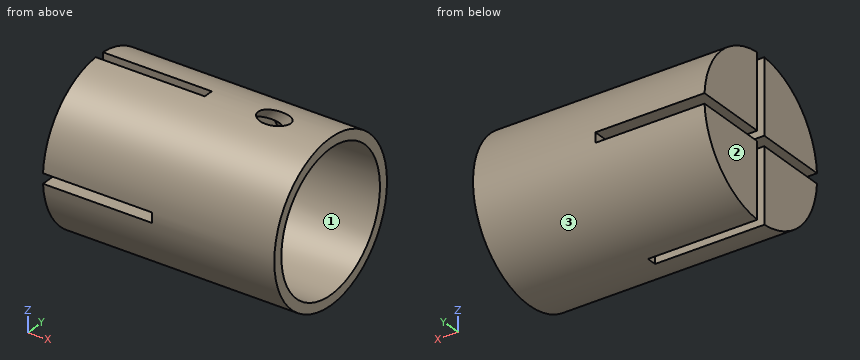
```python
from build123d import *

# Parameters (mm, degrees)
F2_W     = 36.676987372
F2_H     = 3.81
F2_W_2   = 3.81
F2_H_2   = 32.5926636749
F2_W_3   = 35.713012628
F2_H_3   = 39.7973363251
F3_DEPTH = 41.91
F6_R     = 4.445
F7_DEPTH = 76.708


with BuildPart() as f1:
    # F0 (on Front) → F1 (revolve)
    with BuildSketch(Plane.XZ):
        Polygon((-47.0309668349, 30.48), (-47.0309668349, 0), (3.7690331651, 0), (3.7690331651, 26.67), (41.8690331651, 26.67), (41.8690331651, 30.48), align=None)
    revolve(axis=Axis((6.2270945557, 0, 0), (1, 0, 0)))

    # F2 (on face) → F3 (cut)
    with BuildSketch(Plane(origin=(-47.0309668349, 0, 0), x_dir=(0, -1, 0), z_dir=(-1, 0, 0))):
        with Locations((-20.243493686, 0)):
            Rectangle(F2_W, F2_H)
        with Locations((0, 18.2013318375)):
            Rectangle(F2_W_2, F2_H_2)
        Rectangle(F2_W_2, F2_H)
        with Locations((19.761506314, 0)):
            Rectangle(F2_W_3, F2_H)
        with Locations((0, -21.8036681625)):
            Rectangle(F2_W_2, F2_H_3)
    extrude(amount=-F3_DEPTH, mode=Mode.SUBTRACT)

    # F6 (on line) → F7 (cut)
    with BuildSketch(Plane(origin=(66.1142536219, 0, 66.1142536219), x_dir=(0, -1, 0), z_dir=(-0.7071067812, 0, -0.7071067812))):
        with Locations((0, 7.1842048969)):
            Circle(F6_R)
    extrude(amount=F7_DEPTH, mode=Mode.SUBTRACT)


solid = f1.part
```
The model under review builds one solid part; all positions refer to its coordinate system, in mm. Face numbers are marked on the shaded views. Round coordinates to 2 decimals unless told otherwise and drop trailing zeros. Loops run counter-clockwise (first coordinate to the right, second up) from the corner with the lowest first, then second, coordinate; pieces in that order, holes last.
1) Consider section C-C on y = 0. State the section outline as (x, z) points, then the cut area to 3 significant figures.
Values follow:
outline: (-5.12, -30.48) - (41.87, -30.48) - (41.87, -26.67) - (3.77, -26.67) - (3.77, 19.98) - (3.65, 20.1) - (3.77, 20.22) - (3.77, 26.67) - (10.22, 26.67) - (14.03, 30.48) - (-5.12, 30.48) - close; (22.8, 26.67) - (41.87, 26.67) - (41.87, 30.48) - (26.61, 30.48) - close
area: 784 mm2
2) Consider section B-B on x = -11.5. State the section outline as (y, z) points (3 decimals), then the cut area to 3 significant figures.
Values follow:
outline: (-30.42, -1.905) arc R30.48 ccw to (-1.905, -30.42) - (-1.905, -1.905) - close; (-30.42, 1.905) - (-1.905, 1.905) - (-1.905, 30.42) arc R30.48 ccw to start; (1.905, -30.42) arc R30.48 ccw to (30.42, -1.905) - (1.905, -1.905) - close; (1.905, 1.905) - (30.42, 1.905) arc R30.48 ccw to (1.905, 30.42) - close
area: 2,470 mm2
3) Wall thickness on line 1 along Y through (x, z) = (25.5, 0); line 2 along X through (y, z) = (-10.5, -2); line 3 along Z through (x, y) = (18.5, 0): over which ranges is each line inside the solid? List them lowest first.
Values follow:
line 1: y = -30.48 to -26.67, 26.67 to 30.48
line 2: x = -47.03 to 3.77
line 3: z = -30.48 to -26.67
4) Consider section D-D on y = -20. State the section outline as (x, z) points (3 decimals), then the cut area to 3 significant figures.
Values follow:
outline: (-47.031, -23.001) - (41.869, -23.001) - (41.869, -17.643) - (3.769, -17.643) - (3.769, 17.643) - (41.869, 17.643) - (41.869, 23.001) - (-47.031, 23.001) - (-47.031, 1.905) - (-5.121, 1.905) - (-5.121, -1.905) - (-47.031, -1.905) - close
area: 2,590 mm2
5) Consider section A-A on z = 0. State the section outline as (x, y) points.
Values follow:
outline: (-5.12, -30.48) - (41.87, -30.48) - (41.87, -26.67) - (3.77, -26.67) - (3.77, 26.67) - (41.87, 26.67) - (41.87, 30.48) - (-5.12, 30.48) - close
6) The part is to be moulded in two halves that separate along Z. For the marked faces 1, 2 and 3, say which applies: pulls with the +Z half, pulls with the -Z half, needs draft (parallel to the pull), parting line crosses it, or undercut.
Values follow:
face 1: undercut
face 2: needs draft
face 3: parting line crosses it
7) Clearance check with flat-ended pins moving along their axes: P1, Ø6, axis at x = 32, z = 18, coming from the +Y side; P2, Ø6, axis at x = -28, y = 10.5, coming from the -Z side; P3, Ø2, axis at x = 26, z = -7, coming from the +Y side. State where each tip first meets the part, or that it passes through.
Values follow:
P1: stops at y = 26.53
P2: stops at z = -29.54
P3: stops at y = 29.88
